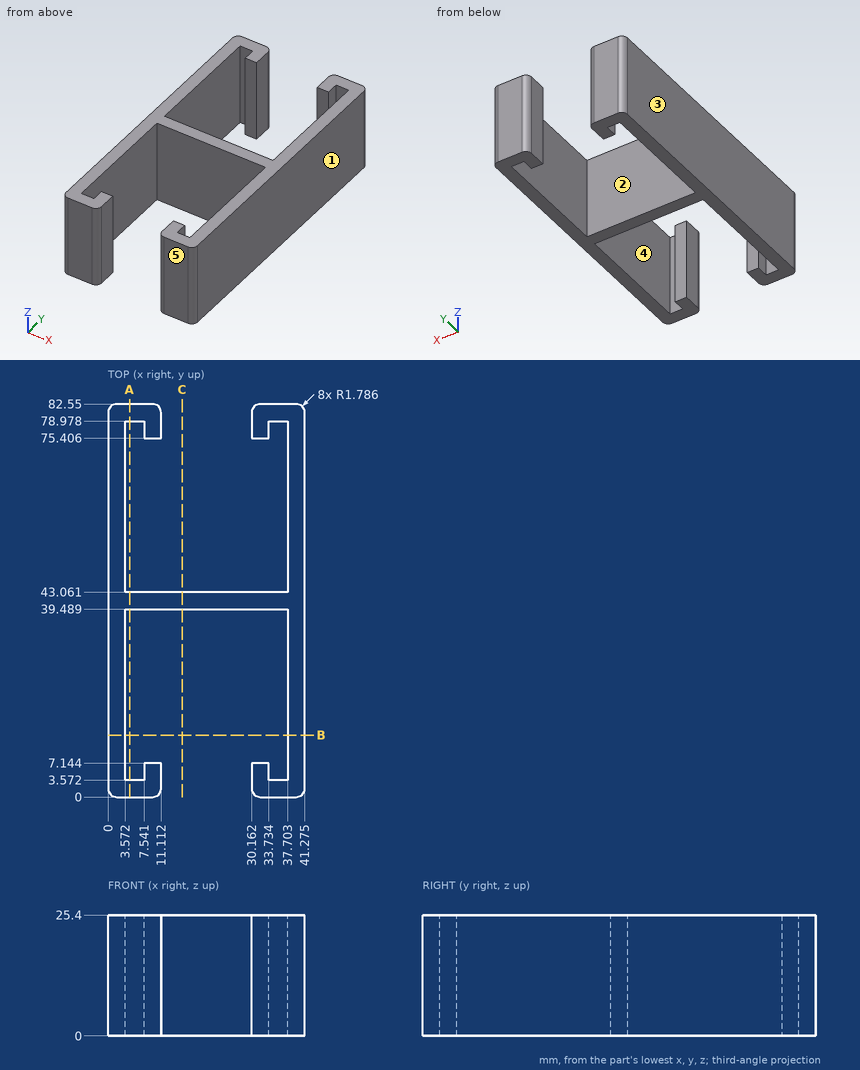
Here's the drawing with two shaded views (mm, measured from the low corner). I have some questions. A direction names the side the tool comes from. Coordinates: 2 decimals unless noted, no trailing zeros. Write each loop counter-clockwise with the first axis right and the second up, starting at its lowest first coordinate (ties: lowest second). Pieces come first, ordered by that corner, then holes. Notation, with made-up numbers: (36.5, -35) -> (46.5, -35) arc R23 cw to (46.5, 0) -> close; hole circle Ø5 at (67.5, 35.5). An arc over 180 degrees is marked (long way). Write item = value, one per line. Start each with the question number.
(1) I need wall thicknesses on line 1 (Y direction, x = 5, z = 13.5); line 2 (X direction, y = 50, z = 14.25) (1 decimal); line 3 (Y direction, x = 9, z = 11). Which ranges of each line are inside material? Lowest first, please. Write a range as [from, to].
(2) We'd pull the mould along X, two halves only. Please class the marked faces 1, 2 and 3: released by +X, released by -X, zero draft, split by the parting line, or undercut.
(3) I want a section at C-C (x = 15.5). Please give me the cut outline in (y, z).
(4) Which directions (+Z, -Z, +X, -X, +Y, -Y) give clear straight access to the entire face, cutting with the end or side of a thin tool? Please do the marked faces 4 and 5.
(5) I want a section at B-B (y = 13). Please give me the cut outline in (x, z) (1 decimal).
(6) Will this pin go through, and if not, where does the flat tip stop? pin 1 (4 mm diameter, centred on x = 21, z = 9, fed in from -Y).
(7) I want a section at A-A (x = 4.5). Please give me the cut outline in (y, z), plus the area to 3 significant figures.
Result set:
q1.line_1 = [0, 3.57], [39.49, 43.06], [78.98, 82.55]
q1.line_2 = [0, 3.6], [37.7, 41.3]
q1.line_3 = [0, 7.14], [39.49, 43.06], [75.41, 82.55]
q2.face_1 = released by +X
q2.face_2 = undercut
q2.face_3 = released by -X
q3.outline = (39.49, 0) -> (43.06, 0) -> (43.06, 25.4) -> (39.49, 25.4) -> close
q4.face_4 = +Z, -Z
q4.face_5 = +Z, -Z, +X, -X, -Y
q5.outline = (0, 0) -> (3.6, 0) -> (3.6, 25.4) -> (0, 25.4) -> close; (37.7, 0) -> (41.3, 0) -> (41.3, 25.4) -> (37.7, 25.4) -> close
q6.pin_1 = 39.49
q7.outline = (0, 0) -> (3.57, 0) -> (3.57, 25.4) -> (0, 25.4) -> close; (39.49, 0) -> (43.06, 0) -> (43.06, 25.4) -> (39.49, 25.4) -> close; (78.98, 0) -> (82.55, 0) -> (82.55, 25.4) -> (78.98, 25.4) -> close
q7.area = 272 mm2
